from build123d import *

# Parameters (mm, degrees)
F0_W     = 22.2654491663
F0_H     = 47.4806427956
F0_R     = 13.033720186
F1_DEPTH = 6


# Not quite as in the source:
# - a feature names something its author has since deleted; it is built from what else it names


with BuildPart() as f1:
    # F0 (on Front) → F1 (new body)
    with BuildSketch(Plane.XZ):
        with BuildLine():
            add(Edge.make_bspline(
                [(111.8640829768, 215), (133.0716213469, 209.4330211779), (135.6474762559, 42.6029998371), (135.8640829768, 10.1536091521)],
                knots=[0, 0, 0, 0, 186.7738886147, 186.7738886147, 186.7738886147, 186.7738886147], degree=3))
            Line((111.8640829768, 215), (91.8640829768, 215))
            Line((91.8640829768, 215), (91.8640829768, 195))
            Line((91.8640829768, 195), (81.8640829768, 195))
            Line((81.8640829768, 195), (81.8640829768, 10))
            Line((81.8640829768, 10), (108.8640829768, 10))
            Line((108.8640829768, 10), (108.8640829768, 5))
            Line((108.8640829768, 5), (135.8640829768, 5))
            Line((135.8640829768, 5), (135.8640829768, 10.1536091521))
        make_face()
        with Locations((103.1980912897, 160.0865775181)):
            Rectangle(F0_W, F0_H, mode=Mode.SUBTRACT)
        with Locations((110.2482031796, 83.6049893333)):
            Circle(F0_R, mode=Mode.SUBTRACT)
        with BuildLine():
            Line((135.8640829768, -0.1536091521), (135.8640829768, 5))
            Line((135.8640829768, 5), (108.8640829768, 5))
            Line((108.8640829768, 5), (108.8640829768, 0))
            Line((108.8640829768, 0), (81.8640829768, 0))
            Line((81.8640829768, 0), (81.8640829768, -185))
            Line((81.8640829768, -185), (91.8640829768, -185))
            Line((91.8640829768, -185), (91.8640829768, -205))
            Line((91.8640829768, -205), (111.8640829768, -205))
            add(Edge.make_bspline(
                [(111.8640829768, -205), (133.0716213469, -199.4330211779), (135.6474762559, -32.6029998371), (135.8640829768, -0.1536091521)],
                knots=[0, 0, 0, 0, 186.7738886147, 186.7738886147, 186.7738886147, 186.7738886147], degree=3))
        make_face()
        with Locations((103.1980912897, -150.0865775181)):
            Rectangle(F0_W, F0_H, mode=Mode.SUBTRACT)
        with Locations((110.2482031796, -73.6049893333)):
            Circle(F0_R, mode=Mode.SUBTRACT)
    extrude(amount=F1_DEPTH)


solid = f1.part
Design review of the part built by this model. Coordinates are the model's own, in mm. Give positions to 0.01 mm unless a question says otherwise; leave off trailing zeros. Order: outer loops, then holes, each group sorted by start corner. A loop starts at its lowest first (then second) coordinate and runs counter-clockwise, first axis right, second up. Notation, with made-up numbers: (39.25, -36) - (74.25, -36) arc R20 ccw to (74.25, -5) - close; hole circle Ø3 at (-3.5, -33.75). An arc over 180 degrees is marked (long way). Write item = value, one per line. Start each with the question number.
Q1. We need section B-B on x = 104. State the section outline as (y, z) points.
Q2. We need section C-C on z = 6.5. State the section outline as (x, y) points.
Q3. To check wall thickness, follow L1, parallel to Z at x = 94.5, y = -1.5; L2, parallel to Z at x = 84, y = -3; L3, parallel to Z at x = 115, y = -5.5. State the ranges of each line that lie inside material, in increasing order. Write a range as from..to.
Q4. Mouldability with a two-part tool opening along Z and no side actions: class faces 1 (the face through (109.2, 0, 7.9)), 2 (the face through (99.91, -2.96, 75.67)) as released by +Z, released by -Z, zero draft, split by the parting line, or undercut.
Q5. Clearance check with flat-ended pins moving along their axes: pin 1 Ø1.8 at (y, z) = (-1.5, 208.5) entering from -X; pin 2 Ø1.5 at (x, z) = (125, 50.5) entering from +Y; pin 3 Ø3 at (x, y) = (85.5, -2.5) entering from -Z. State where each tip first meets the part, or that it passes through.
Q6. We need section A-A on x = 86. State the section outline as (y, z) points.
Q7. We need section D-D on y = -1.25. State how many separate pieces and enclosed holes the cut face has, plus the area to 3 significant figures.
Working result:
q1.outline = (-6, -205) - (0, -205) - (0, -173.83) - (-6, -173.83) - close; (-6, -126.35) - (0, -126.35) - (0, -85.04) - (-6, -85.04) - close; (-6, -62.17) - (0, -62.17) - (0, 0) - (-6, 0) - close; (-6, 10) - (0, 10) - (0, 72.17) - (-6, 72.17) - close; (-6, 95.04) - (0, 95.04) - (0, 136.35) - (-6, 136.35) - close; (-6, 183.83) - (0, 183.83) - (0, 215) - (-6, 215) - close
q2.outline = (108.86, -6) - (135.86, -6) - (135.86, 0) - (108.86, 0) - close
q3.L1 = -205..-173.83, -126.35..0, 10..136.35, 183.83..215
q3.L2 = -185..0, 10..195
q3.L3 = -202.89..-85.74, -61.47..71.47, 95.74..212.89
q4.face_1 = zero draft
q4.face_2 = undercut
q5.pin_1 = 91.86
q5.pin_2 = 0
q5.pin_3 = -185
q6.outline = (-6, -185) - (0, -185) - (0, 0) - (-6, 0) - close; (-6, 10) - (0, 10) - (0, 195) - (-6, 195) - close
q7.separate_pieces = 1
q7.enclosed_holes = 4
q7.area = 16,700 mm²
